For this review, take the finished solid that the model builds, in its own axes (mm). A direction names the side the tool comes from. Coordinates: 2 decimals unless noted, no trailing zeros. Loops run counter-clockwise (first coordinate to the right, second up) from the corner with the lowest first, then second, coordinate; pieces in that order, holes last. Notation, with made-up numbers: (14, 36.5) -> (72, 36.5) arc R29 cw to (72, 60.5) -> close; hole circle Ø6 at (19.5, 15.25). An arc over 180 degrees is marked (long way). Use a Markdown table: item, result.
Autodesk Inventor part; units mm, degrees
ref_plane "YZ Plane" through (0, 0, 0) normal (1, 0, 0) x (0, 1, 0)
ref_plane "XZ Plane" through (0, 0, 0) normal (0, 1, 0) x (-1, 0, 0)
ref_plane "XY Plane" through (0, 0, 0) normal (0, 0, 1) x (1, 0, 0)
sketch "Náčrt2" plane through (0, 0, 0) normal (0, 0, 1) x (1, 0, 0)
  line L0 (0, 0) -> (190, 0)
  line L1 (190, 0) -> (190, -50)
  line L2 (190, -50) -> (0, -50)
  line L3 (0, -50) -> (0, 0)
  dimension "d2" = 190
  dimension "d3" = 50
extrude "Vysunutí2" add sketch "Náčrt2" along normal blind 4
sketch "Náčrt3" plane through (0, 0, 4) normal (0, 0, 1) x (1, 0, 0)
  line L0 (190, 0) -> (0, 0)
  line L1 (0, -50) -> (190, -50)
  line L2 (190, -50) -> (190, 0)
  line L3 (190, 0) -> (0, 0)
  line L4 (0, 0) -> (0, -50)
  line L5 (4, -46) -> (186, -46)
  line L6 (186, -46) -> (186, -4)
  line L7 (186, -4) -> (4, -4)
  line L8 (4, -4) -> (4, -46)
  dimension "d7" = 4
extrude "Vysunutí3" add sketch "Náčrt3" along normal blind 160
sketch "Náčrt4" plane through (0, -50, 0) normal (0, -1, 0) x (1, 0, 0)
  line L0 (4, 164) -> (186, 164)
  line L1 (182, 164) -> (58, 164)
  line L2 (58, 164) -> (58, 64)
  line L3 (58, 64) -> (182, 64)
  line L4 (182, 64) -> (182, 164)
  line L5 (190, 0) -> (190, 164)
  point P0 (0, 0)
  dimension "d10" = 8
  dimension "d11" = 100
  dimension "d12" = 124
extrude "Vysunutí4" cut sketch "Náčrt4" against normal blind 10
sketch "Náčrt5" plane through (4, -4, 4) normal (0, -1, 0) x (1, 0, 0)
  line L0 (54, 60) -> (54, 160)
  line L1 (178, 60) -> (54, 60)
  circle A0 centre (151, 125) radius 4
  circle A1 centre (71, 125) radius 4
  line L2 (186, -4) -> (186, 160)
  line L3 (0, 160) -> (182, 160)
  point P0 (-4, -4)
  dimension "d15" = 8
  dimension "d16" = 8
  dimension "d17" = 35
  dimension "d18" = 80
  dimension "d19" = 35
  dimension "d20" = 35
extrude "Vysunutí5" cut sketch "Náčrt5" against normal blind 10
sketch "Náčrt6" plane through (4, -46, 4) normal (0, 1, 0) x (1, 0, 0)
  line L0 (-4, 4) -> (186, 4)
  line L1 (-4, 4) -> (-4, -160)
  line L2 (178, -160) -> (178, -60)
  line L3 (178, -60) -> (54, -60)
  line L4 (54, -60) -> (54, -160)
  line L5 (-4, -160) -> (54, -160)
  line L6 (-4, 4) -> (-4, -160)
  line L7 (-4, 4) -> (186, 4)
  line L8 (186, 4) -> (186, -160)
  line L9 (178, -160) -> (186, -160)
extrude "Vysunutí6" add sketch "Náčrt6" along normal blind 3
sketch "Náčrt7" plane through (0, 0, 164) normal (0, 0, 1) x (1, 0, 0)
  line L0 (184.5, -47) -> (4, -47)
  line L1 (4, -47) -> (4, -45)
  line L2 (4, -45) -> (184.5, -45)
  line L3 (184.5, -45) -> (184.5, -47)
  line L4 (182, -43) -> (182, -50)
  line L5 (182, -50) -> (190, -50)
  point P0 (0, 0)
  dimension "d25" = 2.5
  dimension "d26" = 2
  dimension "d27" = 3
  dimension "d28" = 180.5
extrude "Vysunutí7" cut sketch "Náčrt7" against normal blind 105
sketch "Náčrt8" plane through (4, -43, 4) normal (0, 1, 0) x (1, 0, 0)
  line L0 (54, -160) -> (54, -60)
  line L1 (0, -160) -> (54, -160)
  line L2 (54, -160) -> (0, -160)
  line L3 (0, -160) -> (0, -60)
  line L4 (0, -60) -> (54, -60)
  line L5 (54, -60) -> (54, -160)
  point P0 (-4, 4)
  point P1 (54, -60)
  dimension "d31" = 54
  dimension "d32" = 100
extrude "Vysunutí8" cut sketch "Náčrt8" against normal up to surface (4 mm away)
sketch "Náčrt9" plane through (4, -43, 4) normal (0, 1, 0) x (1, 0, 0)
  line L0 (54, -60) -> (54, -160)
  line L1 (0, 0) -> (54, 0)
  line L2 (54, 0) -> (54, -60)
  line L3 (54, -60) -> (0, -60)
  line L4 (0, -60) -> (0, 0)
  point P0 (-4, 4)
  dimension "d35" = 54
extrude "Vysunutí9" cut sketch "Náčrt9" against normal blind 4
sketch "Náčrt10" plane through (190, -50, 0) normal (1, 0, 0) x (0, 0, -1)
  circle A0 centre (-149, 25) radius 2.5
  line L0 (0, 0) -> (-164, 0)
  line L1 (-164, 0) -> (-164, 50)
  point P0 (0, 50)
  dimension "d38" = 5
  dimension "d39" = 25
  dimension "d40" = 15
extrude "Vysunutí10" cut sketch "Náčrt10" against normal through all
sketch "Náčrt11" plane through (0, 0, 4) normal (0, 0, 1) x (1, 0, 0)
  circle A0 centre (25.2842, -14.6015) radius 2.5
  circle A1 centre (35.2842, -14.6015) radius 2.5
  circle A2 centre (45.2842, -14.6015) radius 2.5
  circle A3 centre (31.1056, -24.6015) radius 2.5
  circle A4 centre (41.1056, -24.6015) radius 2.5
  circle A5 centre (36.7049, -34.6015) radius 2.5
  line L0 (25.2842, -14.6015) -> (59.2692, -14.6015) construction
  line L1 (31.1056, -24.6015) -> (52.5835, -24.6015) construction
  point P0 (0, 0)
  dimension "d43" = 5
  dimension "d44" = 5
  dimension "d45" = 5
  dimension "d46" = 5
  dimension "d47" = 5
  dimension "d48" = 5
  dimension "d49" = 10
  dimension "d50" = 10
  dimension "d51" = 10
  dimension "d52" = 10
  dimension "d53" = 10
extrude "Vysunutí11" cut sketch "Náčrt11" against normal through all
pattern_linear "Obdélníkové pole1" count 3 spacing 55 along (1, 0, 0) of "Vysunutí11"
properties part number "krab2"
(1) Take a section at C-C on y = -6.5. Write out the cut boundary in (x, z).
Found:
| item | result |
|---|---|
| outline | (0, 0) -> (190, 0) -> (190, 164) -> (186, 164) -> (186, 4) -> (4, 4) -> (4, 164) -> (0, 164) -> close |
(2) Take a section at D-D on x = 114. Write out the cut boundary in (y, z), plus the area to 3 significant figures.
Found:
| item | result |
|---|---|
| outline | (-50, 0) -> (0, 0) -> (0, 164) -> (-4, 164) -> (-4, 4) -> (-43, 4) -> (-43, 64) -> (-45, 64) -> (-45, 59) -> (-47, 59) -> (-47, 64) -> (-50, 64) -> close |
| area | 1,250 mm^2 |
(3) For line 1 along Y through (x, z) = (8, 115.5); line 2 along Z through (x, y) = (155, -1.45); line 3 along X through (y, z) = (-17, 137), list the stretches that pass through material, from the lowest coordinate up.
Found:
| item | result |
|---|---|
| line 1 | y = -50 to -47, -4 to 0 |
| line 2 | z = 0 to 125, 133 to 164 |
| line 3 | x = 0 to 4, 186 to 190 |
(4) Take a section at A-A on x = 75. Write out the cut boundary in (y, z).
Found:
| item | result |
|---|---|
| outline | (-50, 0) -> (0, 0) -> (0, 125) -> (-4, 125) -> (-4, 4) -> (-43, 4) -> (-43, 64) -> (-45, 64) -> (-45, 59) -> (-47, 59) -> (-47, 64) -> (-50, 64) -> close; (-4, 133) -> (0, 133) -> (0, 164) -> (-4, 164) -> close |
(5) Mouldability with a two-part tool opening along X and no side actions: class faces 3 (the face through (97.787, -14.492, 2.028)), 4 (the face through (88, -3, 164)), 5 (the face through (0, -25, 81)) as pulls with the +X half, pulls with the -X half, needs draft (parallel to the pull), parting line crosses it, or undercut.
Found:
| item | result |
|---|---|
| face 3 | undercut |
| face 4 | needs draft |
| face 5 | pulls with the -X half |
(6) Take a section at B-B on z = 149. Write out the cut boundary in (x, y).
Found:
| item | result |
|---|---|
| outline | (0, -50) -> (58, -50) -> (58, -47) -> (4, -47) -> (4, -27.5) -> (0, -27.5) -> close; (0, -22.5) -> (4, -22.5) -> (4, -4) -> (186, -4) -> (186, -22.5) -> (190, -22.5) -> (190, 0) -> (0, 0) -> close; (182, -50) -> (190, -50) -> (190, -27.5) -> (186, -27.5) -> (186, -43) -> (182, -43) -> (182, -45) -> (184.5, -45) -> (184.5, -47) -> (182, -47) -> close |
(7) For pin 1 Ø6.5 at (x, y) = (146.7, -34.6) entering from +Z; pin 2 Ø3 at (x, z) = (132, 129) entering from -Y, all flat-tipped, find the tip position at first contact; note any pin that passes through.
Found:
| item | result |
|---|---|
| pin 1 | stops at z = 4 |
| pin 2 | stops at y = -4 |
(8) For faces 1 (the face through (96, -4, 83)), 2 (the face through (142.787, -14.492, 2.028)), list the 3-axis set-ups (+Z, -Z, +X, -X, +Y, -Y) from which the entire face can be reached by the end or side of a thin tool; tool diameter is ignored.
Found:
| item | result |
|---|---|
| face 1 | +Z |
| face 2 | +Z, -Z |
